Autodesk Inventor part; units mm, degrees
ref_plane "Start plane" through (0, 0, -17.5) normal (0, 0, 1) x (1, 0, 0)
ref_plane "End plane" through (0, 0, 447.5) normal (0, 0, 1) x (1, 0, 0)
ref_plane "Work Plane4" through (17.5, 0, 447.5) normal (-0.7071, 0, 0.7071) x (0.7071, 0, 0.7071)
ref_plane "Start plane" through (0, 0, -17.5) normal (0, 0, 1) x (1, 0, 0)
ref_plane "End plane" through (0, 0, 447.5) normal (0, 0, 1) x (1, 0, 0)
sketch "Sketch" plane through (0, 0, 0) normal (0, 0, 1) x (1, 0, 0)
  line L0 (-17.5, -11.5) -> (-17.5, 11.5)
  line L1 (-11.5, 17.5) -> (11.5, 17.5)
  line L2 (17.5, 11.5) -> (17.5, -11.5)
  line L3 (11.5, -17.5) -> (-11.5, -17.5)
  arc A0 (-17.5, -11.5) -> (-11.5, -17.5) centre (-11.5, -11.5) ccw
  arc A1 (-11.5, 17.5) -> (-17.5, 11.5) centre (-11.5, 11.5) ccw
  arc A2 (17.5, 11.5) -> (11.5, 17.5) centre (11.5, 11.5) ccw
  arc A3 (11.5, -17.5) -> (17.5, -11.5) centre (11.5, -11.5) ccw
  arc A4 (-11.5, 14.5) -> (-14.5, 11.5) centre (-11.5, 11.5) ccw
  line L4 (-11.5, 14.5) -> (11.5, 14.5)
  arc A5 (14.5, 11.5) -> (11.5, 14.5) centre (11.5, 11.5) ccw
  line L5 (14.5, 11.5) -> (14.5, -11.5)
  arc A6 (11.5, -14.5) -> (14.5, -11.5) centre (11.5, -11.5) ccw
  line L6 (11.5, -14.5) -> (-11.5, -14.5)
  arc A7 (-14.5, -11.5) -> (-11.5, -14.5) centre (-11.5, -11.5) ccw
  line L7 (-14.5, -11.5) -> (-14.5, 11.5)
  line L8 (0, 25.4278) -> (0, -25.4278) construction
  line L9 (-25.4278, 0) -> (25.4278, 0) construction
  dimension "d7" = 6
  dimension "d10" = 35
  dimension "d11" = 35
  dimension "d12" = 3
  dimension "d15" = 17.5
  dimension "d16" = 17.5
extrude "Body" add sketch "Sketch" along normal up to surface (465 mm away) from surface at -17.5
sketch "Sketch3" plane through (0, 0, 0) normal (0, 0, 1) x (1, 0, 0)
  line L0 (0, 0) -> (10, 0)
ref_plane "Work Plane3" through (0, 0, 0) normal (0, -1, 0) x (1, 0, 0)
sketch "Sketch4" plane through (0, 0, 0) normal (0, -1, 0) x (1, 0, 0)
  line L0 (-2, -17.5) -> (12, -17.5)
  line L1 (-2, 447.5) -> (12, 447.5)
  dimension "d18" = 465
ref_plane "Work Plane4" through (17.5, 0, 447.5) normal (-0.7071, 0, 0.7071) x (0.7071, 0, 0.7071)
split "Split1" plane through (17.5, 0, 447.5) removes the side toward (-0.7071, 0, 0.7071)
ref_plane "Work Plane5" through (17.5, 0, -17.5) normal (-0.7071, 0, -0.7071) x (-0.7071, 0, 0.7071)
split "Split2" plane through (17.5, 0, -17.5) removes the side toward (-0.7071, 0, -0.7071)
ref_plane "Work Plane6" through (-730, 0, 215) normal (1, 0, 0) x (0, 0, -1)
ref_plane "Work Plane7" through (0, 0, 215) normal (1, 0, 0) x (0, 0, -1)
ref_plane "Work Plane8" through (-365, 0, 215) normal (1, 0, 0) x (0, 0, -1)
sketch "Sketch5" plane through (-365, 0, 215) normal (1, 0, 0) x (0, 0, -1)
  arc A0 (-17.5, -12.5) -> (-12.5, -17.5) centre (-12.5, -12.5) ccw
  line L0 (-17.5, -12.5) -> (-17.5, 12.5)
  arc A1 (-12.5, 17.5) -> (-17.5, 12.5) centre (-12.5, 12.5) ccw
  line L1 (-12.5, 17.5) -> (12.5, 17.5)
  arc A2 (17.5, 12.5) -> (12.5, 17.5) centre (12.5, 12.5) ccw
  line L2 (17.5, 12.5) -> (17.5, -12.5)
  arc A3 (12.5, -17.5) -> (17.5, -12.5) centre (12.5, -12.5) ccw
  line L3 (12.5, -17.5) -> (-12.5, -17.5)
  arc A4 (-12.5, 15) -> (-15, 12.5) centre (-12.5, 12.5) ccw
  line L4 (-12.5, 15) -> (12.5, 15)
  arc A5 (15, 12.5) -> (12.5, 15) centre (12.5, 12.5) ccw
  line L5 (15, 12.5) -> (15, -12.5)
  arc A6 (12.5, -15) -> (15, -12.5) centre (12.5, -12.5) ccw
  line L6 (12.5, -15) -> (-12.5, -15)
  arc A7 (-15, -12.5) -> (-12.5, -15) centre (-12.5, -12.5) ccw
  line L7 (-15, -12.5) -> (-15, 12.5)
extrude "Extrusion2" cut sketch "Sketch5" along normal up to surface (730 mm away) from surface at -365 contours L0 A1 L1 A2 L2 A3 L3 A0 | L4 A5 L5 A6 L6 A7 L7 A4
equation "\"d7\" = G_IR"
equation "\"d10\" = G_H"
equation "\"d11\" = G_W"
equation "\"d12\" = G_T"
equation "\"d15\" = 0.5 * d10"
equation "\"d16\" = 0.5 * d11"
equation "\"d3\" = G_L"
equation "\"G_W\" = 35"
equation "\"G_H\" = 35"
equation "\"G_T\" = 3"
equation "\"G_IR\" = 6"
equation "\"G_L\" = d18"
equation "\"G_OFFSET_START\" = 17.5"
equation "\"G_OFFSET_END\" = 17.5"
equation "\"d13\" = -G_OFFSET_START"
equation "\"d14\" = G_OFFSET_END + B_L"
properties part number "AS 1163 - C350L0 35x35x3.0 SHS - 465" material "Steel, Mild"
Source: CAD feature listing. Evaluate the final solid. Frame: model axes, mm. A direction names the side the tool comes from. Coordinates: 2 decimals unless noted, no trailing zeros. Loops run counter-clockwise (first coordinate to the right, second up) from the corner with the lowest first, then second, coordinate; pieces in that order, holes last. Notation, with made-up numbers: M 61.25,-39.5 L 73.25,-39.5 A14 cw 73.25,-29.5 Z; hole C -38,-22 d2. An arc over 180 degrees is marked long. Answer in a Markdown table with one row per item.
Q1. Draft query along Y for faces 1 (the flat face through (0.2, -14.5, 211.8)), 2 (the flat face through (0, 15, 430)), 3 (the flat face through (2, 14.5, 212)), 4 (the flat face through (2, 17.5, 212)). Return one class per face: pulls with the +Y half, pulls with the -Y half, needs draft (parallel to the pull), parting line crosses it, or undercut.
Answers below:
| item | result |
|---|---|
| face 1 | undercut |
| face 2 | needs draft |
| face 3 | undercut |
| face 4 | pulls with the +Y half |
Q2. Ray query, probe 1 along Y at (x, z) = (9.5, 299); probe 2 along Y at (x, z) = (-13, 306.5). Return the intervals inside material, ascending. Write a range as from..to.
Answers below:
| item | result |
|---|---|
| probe 1 | y = -17.5..-14.5, 14.5..17.5 |
| probe 2 | y = -17.31..-14.1, 14.1..17.31 |
Q3. Section B-B on z = 338. Return the cut outline in (x, y).
Answers below:
| item | result |
|---|---|
| outline | M -17.5,-11.5 A6 ccw -11.5,-17.5 L 11.5,-17.5 A6 ccw 17.5,-11.5 L 17.5,11.5 A6 ccw 11.5,17.5 L -11.5,17.5 A6 ccw -17.5,11.5 Z; hole M -14.5,-11.5 A3 ccw -11.5,-14.5 L 11.5,-14.5 A3 ccw 14.5,-11.5 L 14.5,11.5 A3 ccw 11.5,14.5 L -11.5,14.5 A3 ccw -14.5,11.5 Z |
Q4. First-contact query: pin 1 (5 mm diameter, centred on x = -10, y = 4, fed in from +Z); pin 2 (1.5 mm diameter, centred on y = 15.5, z = 207, fed in from -X); pin 3 (1.6 mm diameter, centred on x = -16, y = 0.5, fed in from -Z); pin 4 (1.6 mm diameter, centred on x = -15.5, y = 2, fed in from +Z). Flat tips, straight axial feed; report the tip coordinate or a pass-through.
Answers below:
| item | result |
|---|---|
| pin 1 | passes through |
| pin 2 | stops at x = 0 |
| pin 3 | stops at z = 15.2 |
| pin 4 | stops at z = 415.3 |
Q5. Set-up query: faces 5 (the flat face through (17.5, 0, 212)), 6 (the flat face through (-14.5, 0, 323)). Return all of +Z, -Z, +X, -X, +Y, -Y with unobstructed straight access to the full face (end or side cutting, diameter ignored); none if empty.
Answers below:
| item | result |
|---|---|
| face 5 | +Z, -Z, +X, +Y, -Y |
| face 6 | +Z, -Z |
Q6. Section A-A on y = -1. Return the cut outline in (x, z), plus the area to 4 significant figures.
Answers below:
| item | result |
|---|---|
| outline | M -17.5,17.5 L -14.5,14.5 L -14.5,197.5 L -17.5,197.5 Z; M -17.5,232.5 L -14.5,232.5 L -14.5,415.5 L -17.5,412.5 Z; M 14.5,-14.5 L 17.5,-17.5 L 17.5,447.5 L 14.5,444.5 Z |
| area | 2,475 mm^2 |
